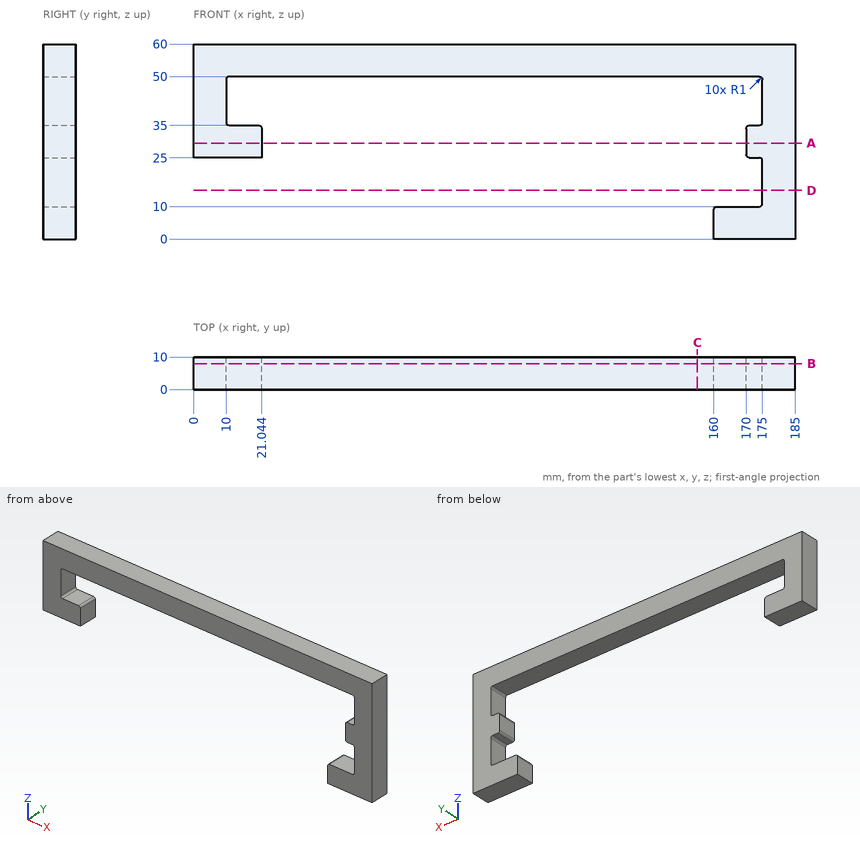
Verification items for this drawing (mm, ordinates from the low corner). Round coordinates to 2 decimals unless told otherwise and drop trailing zeros. Loops run counter-clockwise (first coordinate to the right, second up) from the corner with the lowest first, then second, coordinate; pieces in that order, holes last. Notation, with made-up numbers: M -40,25 L -19,25 A30 cw -19,49 Z; hole C 11.5,24 d9. An arc over 180 degrees is marked long. Answer as a JSON object with one key per item and string values.
1. Gauge pin test, flat ends, axial feed: P1, Ø3, axis at y = 4.5, z = 15.5, coming from the -X side; P2, Ø2.5, axis at x = 172.5, y = 5.5, coming from the -Z side; P3, Ø4.5, axis at y = 6.5, z = 3, coming from the -X side; P4, Ø3, axis at x = 48.5, y = 1, coming from the -Z side. Record the tip position at first contact, or that the pin passes through.
Reply:
{"P1": "stops at x = 175", "P2": "stops at z = 0", "P3": "stops at x = 160", "P4": "stops at z = 50"}
2. Section check D-D (z = 15). Record the boundary of the cut face in (x, y).
Reply:
{"outline": "M 175,0 L 185,0 L 185,10 L 175,10 Z"}
3. Scan lines: line 1 (X direction, y = 3.25, z = 37.5); line 2 (X direction, y = 3.25, z = 31); line 3 (X direction, y = 4, z = 4). Record each from-to range of solid material in increasing order.
Reply:
{"line 1": "x = 0 to 10, 175 to 185", "line 2": "x = 0 to 21.04, 170 to 185", "line 3": "x = 160 to 185"}
4. Section check B-B (y = 8). Record the boundary of the cut face in (x, z).
Reply:
{"outline": "M 0,25 L 21.04,25 L 21.04,34 A1 ccw 20.04,35 L 11,35 A1 cw 10,36 L 10,49 A1 cw 11,50 L 174,50 A1 cw 175,49 L 175,36 A1 cw 174,35 L 171,35 A1 ccw 170,34 L 170,26 A1 ccw 171,25 L 174,25 A1 cw 175,24 L 175,11 A1 cw 174,10 L 161,10 A1 ccw 160,9 L 160,0 L 185,0 L 185,60 L 0,60 Z"}
5. Section check A-A (z = 29.5). Record the boundary of the cut face in (x, y).
Reply:
{"outline": "M 0,0 L 21.04,0 L 21.04,10 L 0,10 Z; M 170,0 L 185,0 L 185,10 L 170,10 Z"}
6. Section check C-C (x = 155). Record the boundary of the cut face in (y, z).
Reply:
{"outline": "M 0,50 L 10,50 L 10,60 L 0,60 Z"}
